from build123d import *

# Parameters (mm, degrees)
SKETCH_1_W                       = 400
SKETCH_1_H                       = 135
SKETCH_1_R                       = 3
SM_BASE_FLANGE_1_DEPTH           = 0.7
SM_EDGE_FLANGE_1_STRIP_W         = 3.2
SM_EDGE_FLANGE_1_STRIP_H         = 0.7
SM_EDGE_FLANGE_1_STRIP_CUT_DEPTH = 400
SM_EDGE_FLANGE_1_DEPTH           = 400


# Sheet-metal steps are written as plain solids
with BuildPart() as part:
    # Sketch 1 → 基体-法兰1 (new body)
    with BuildSketch(Plane(origin=(0, 0, 0), x_dir=(1, 0, 0), z_dir=(0, 1, 0))):
        Rectangle(SKETCH_1_W, SKETCH_1_H)
        with Locations(Location((-194.5, -60.5, 0), (0, 0, 270))):
            Circle(SKETCH_1_R, mode=Mode.SUBTRACT)
        with Locations(Location((-194.5, -10.5, 0), (0, 0, 270))):
            Circle(SKETCH_1_R, mode=Mode.SUBTRACT)
        with Locations(Location((-194.5, -0.5, 0), (0, 0, 270))):
            Circle(SKETCH_1_R, mode=Mode.SUBTRACT)
        with Locations(Location((-194.5, 49.5, 0), (0, 0, 270))):
            Circle(SKETCH_1_R, mode=Mode.SUBTRACT)
        with Locations(Location((0, -10.5, 0), (0, 0, 270))):
            Circle(SKETCH_1_R, mode=Mode.SUBTRACT)
        with Locations(Location((0, -0.5, 0), (0, 0, 270))):
            Circle(SKETCH_1_R, mode=Mode.SUBTRACT)
        with Locations(Location((194.5, -60.5, 0), (0, 0, 90))):
            Circle(SKETCH_1_R, mode=Mode.SUBTRACT)
        with Locations(Location((194.5, -10.5, 0), (0, 0, 90))):
            Circle(SKETCH_1_R, mode=Mode.SUBTRACT)
        with Locations(Location((194.5, -0.5, 0), (0, 0, 90))):
            Circle(SKETCH_1_R, mode=Mode.SUBTRACT)
        with Locations(Location((194.5, 49.5, 0), (0, 0, 90))):
            Circle(SKETCH_1_R, mode=Mode.SUBTRACT)
    extrude(amount=-SM_BASE_FLANGE_1_DEPTH)

    # 边线-法兰1 strip (across the edge) → 边线-法兰1 strip cut (cut)
    with BuildSketch(Plane(origin=(-200, -0.7, -67.5), x_dir=(0, 0, 1), z_dir=(1, 0, 0))):
        with Locations((-0.7, -0.35)):
            Rectangle(SM_EDGE_FLANGE_1_STRIP_W, SM_EDGE_FLANGE_1_STRIP_H)
    extrude(amount=SM_EDGE_FLANGE_1_STRIP_CUT_DEPTH, mode=Mode.SUBTRACT)

    # 边线-法兰1 section (across the edge) → 边线-法兰1 (add)
    with BuildSketch(Plane(origin=(-200, -0.7, -67.5), x_dir=(0, 0, 1), z_dir=(1, 0, 0))):
        with BuildLine():
            Line((0, 0.2), (0, 3.3))
            Line((0, 3.3), (0.7, 3.3))
            Line((0.7, 3.3), (0.7, 0.2))
            ThreePointArc((0.7, 0.2), (0.758578644, 0.058578644), (0.9, 0))
            Line((0.9, 0), (0.9, -0.7))
            ThreePointArc((0.9, -0.7), (0.263603897, -0.436396103), (0, 0.2))
        make_face()
    extrude(amount=SM_EDGE_FLANGE_1_DEPTH)


solid = part.part
For this review, take the finished solid that the model builds, in its own axes (mm). A direction names the side the tool comes from. Give positions to 0.01 mm unless a question says otherwise; leave off trailing zeros. Order: outer loops, then holes, each group sorted by start corner. A loop starts at its lowest first (then second) coordinate and runs counter-clockwise, first axis right, second up. Notation, with made-up numbers: M 54.5,28 L 92.5,28 A28 cw 92.5,60 Z; hole C -25.5,12.25 d11. An arc over 180 degrees is marked long. Answer in a Markdown table with one row per item. Add a question column.
(1) Consider section C-C on y = -2. State the section outline as (x, z) points, and give its area (3 significant figures).
(2) Consider section B-B on z = -39. State the section outline as (x, y) points, and give its area (3 significant figures).
(3) For faces 1 (the face through (-3, -0.7, -15)), 2 (the face through (-3, 0, -15)), list the 3-axis set-ups (+Z, -Z, +X, -X, +Y, -Y) from which the entire face can be reached by the end or side of a thin tool; tool diameter is ignored.
(4) Wall thickness on probe 1 along X at (y, z) = (-0.2, 10.5); probe 2 along X at (y, z) = (-0.15, -49.5); probe 3 along Z at (x, y) = (-194.5, -0.55): over which ranges is each line inside the solid? List them lowest first. Write a range as [from, to].
(5) For pin 1 (2 mm diameter, centred on y = -3.5, z = 52, fed in from +X); pin 2 (9.5 mm diameter, centred on x = -194.5, z = -49.5, fed in from +Y); pin 3 (9.5 mm diameter, centred on x = -194.5, z = 0.5, fed in from -Y); pin 4 (0.9 mm diameter, centred on x = -72, y = -2.5, fed in from +Z), all flat-tipped, find the tip position at first contact; note any pin that passes through.
(6) Consider section A-A on x = -126. State the section outline as (y, z) points, and give its area (3 significant figures).
Evaluation:
| question | item | result |
|---|---|---|
| 1 | outline | M -200,-67.5 L 200,-67.5 L 200,-66.8 L -200,-66.8 Z |
| 1 | area | 280 mm^2 |
| 2 | outline | M -200,-0.7 L 200,-0.7 L 200,0 L -200,0 Z |
| 2 | area | 280 mm^2 |
| 3 | face 1 | +Z, +X, -X, -Y |
| 3 | face 2 | +Z, -Z, +X, -X, +Y |
| 4 | probe 1 | x = [-200, -197.5], [-191.5, -3], [3, 191.5], [197.5, 200] |
| 4 | probe 2 | x = [-200, -197.5], [-191.5, 191.5], [197.5, 200] |
| 4 | probe 3 | z = [-67.43, -52.5], [-46.5, -2.5], [3.5, 7.5], [13.5, 57.5], [63.5, 67.5] |
| 5 | pin 1 | passes through |
| 5 | pin 2 | stops at y = 0 |
| 5 | pin 3 | stops at y = -0.7 |
| 5 | pin 4 | stops at z = -66.8 |
| 6 | outline | M -4,-67.5 L -0.9,-67.5 A0.9 ccw 0,-66.6 L 0,67.5 L -0.7,67.5 L -0.7,-66.6 A0.2 cw -0.9,-66.8 L -4,-66.8 Z |
| 6 | area | 96.6 mm^2 |
